The listing builds one solid part. Answer for the finished solid, in the listing's coordinates (mm). Give positions to 0.01 mm unless a question says otherwise; leave off trailing zeros. Write each loop counter-clockwise with the first axis right and the second up, starting at its lowest first coordinate (ties: lowest second). Pieces come first, ordered by that corner, then holes. Notation, with made-up numbers: M 14.25,30 L 33.25,30 A27 cw 33.25,58 Z; hole C 26,-19 d4. An arc over 180 degrees is marked long. Return JSON: item names as keys, results as strings.
from build123d import *

# Parameters (mm, degrees)
SKETCH086_W   = 102
SKETCH086_H   = 95
PAD035_DEPTH  = 1.6
SKETCH087_R   = 3
HOLE010_DEPTH = 25
FILLET044_R   = 6.35


with BuildPart() as part:
    # Sketch086 → Pad035 (new body)
    with BuildSketch(Plane.XY):
        Rectangle(SKETCH086_W, SKETCH086_H)
    extrude(amount=PAD035_DEPTH)

    # Sketch087 (on Face6 of Pad035) → Hole010 (cut)
    with BuildSketch(Plane.XY.offset(1.6)):
        with Locations((43.38, 39.88)):
            Circle(SKETCH087_R)
        with Locations((43.38, -40.12)):
            Circle(SKETCH087_R)
        with Locations((-42.97, -40.12)):
            Circle(SKETCH087_R)
        with Locations((-42.97, 39.88)):
            Circle(SKETCH087_R)
    extrude(amount=-HOLE010_DEPTH, mode=Mode.SUBTRACT)

    # Fillet044
    fillet044_edges = [part.edges().sort_by_distance(p)[0] for p in [
        (-51, -47.5, 0.8),
        (-51, 47.5, 0.8),
        (51, 47.5, 0.8),
        (51, -47.5, 0.8),
    ]]
    fillet(fillet044_edges, radius=FILLET044_R)


solid = part.part
Item 1: A cutting plane is placed at C-C, the plane y = 39.88. Write down the section's boundary in (x, z), plus the area to 3 significant figures.
Geometry results:
{"outline": "M -51,0 L -45.97,0 L -45.97,1.6 L -51,1.6 Z; M -39.97,0 L 40.38,0 L 40.38,1.6 L -39.97,1.6 Z; M 46.38,0 L 51,0 L 51,1.6 L 46.38,1.6 Z", "area": "144 mm2"}
Item 2: A cutting plane is placed at B-B, the plane z = 0.35. Write down the section's boundary in (x, y).
Geometry results:
{"outline": "M -51,-41.15 A6.35 ccw -44.65,-47.5 L 44.65,-47.5 A6.35 ccw 51,-41.15 L 51,41.15 A6.35 ccw 44.65,47.5 L -44.65,47.5 A6.35 ccw -51,41.15 Z; hole C -42.97,-40.12 d6; hole C -42.97,39.88 d6; hole C 43.38,-40.12 d6; hole C 43.38,39.88 d6"}
Item 3: Find the intervals of material crossed by line 1 (Y direction, x = 43.38, z = 0.3); line 2 (X direction, y = -39, z = 0.1); line 3 (X direction, y = 42, z = 0.55), in increasing order.
Geometry results:
{"line 1": "y = -47.5 to -43.12, -37.12 to 36.88, 42.88 to 47.5", "line 2": "x = -51 to -45.75, -40.19 to 40.6, 46.16 to 51", "line 3": "x = -50.94 to -45.09, -40.85 to 41.26, 45.5 to 50.94"}
Item 4: A cutting plane is placed at A-A, the plane x = -42.97. Write down the section's boundary in (y, z).
Geometry results:
{"outline": "M -47.5,0 L -43.12,0 L -43.12,1.6 L -47.5,1.6 Z; M -37.12,0 L 36.88,0 L 36.88,1.6 L -37.12,1.6 Z; M 42.88,0 L 47.5,0 L 47.5,1.6 L 42.88,1.6 Z"}
Item 5: Determine the mould class of faces 1 (the flat face through (-1, 1, 0)), 2 (the cylindrical face through (40.383, -39.988, 0.811)), 3 (the cylindrical face through (-49.19, -45.59, 0.81)), 4 (the cylindrical face through (-40.11, 40.78, 0.81)) for opening direction X: +X half, -X half, draft (parallel to the pull), parting line (faces both ways), or undercut.
Geometry results:
{"face 1": "draft", "face 2": "undercut", "face 3": "-X half", "face 4": "undercut"}
